```python
from build123d import *

# Parameters (mm, degrees)
SKETCH_1_R      = 1.2
EXTRUDE_1_DEPTH = 15
SKETCH_1_3_R    = 1.2
EXTRUDE_2_DEPTH = 15


with BuildPart() as part:
    # Sketch 1 → Extrude 1 (new body)
    with BuildSketch(Plane(origin=(0, 0, 0), x_dir=(1, 0, 0), z_dir=(0, 1, 0))):
        with BuildLine():
            Line((6.05, 2.5), (-6.05, 2.5))
            ThreePointArc((-6.05, 2.5), (-4.282233047, 1.767766953), (-3.55, 0))
            ThreePointArc((-3.55, 0), (-4.282233047, -1.767766953), (-6.05, -2.5))
            Line((-6.05, -2.5), (6.05, -2.5))
            ThreePointArc((6.05, -2.5), (8.55, 0), (6.05, 2.5))
        make_face()
        with Locations((6.05, 0)):
            Circle(SKETCH_1_R, mode=Mode.SUBTRACT)
        with BuildLine():
            ThreePointArc((-3.55, 0), (-4.282233047, 1.767766953), (-6.05, 2.5))
            ThreePointArc((-6.05, 2.5), (-8.55, 0), (-6.05, -2.5))
            ThreePointArc((-6.05, -2.5), (-4.282233047, -1.767766953), (-3.55, 0))
        make_face()
        with Locations((-6.05, 0)):
            Circle(SKETCH_1_R, mode=Mode.SUBTRACT)
    extrude(amount=EXTRUDE_1_DEPTH)

    # Sketch 1_3 → Extrude 2 (add)
    with BuildSketch(Plane(origin=(0, 0, 0), x_dir=(1, 0, 0), z_dir=(0, 1, 0))):
        with BuildLine():
            ThreePointArc((-3.55, 0), (-4.282233047, 1.767766953), (-6.05, 2.5))
            ThreePointArc((-6.05, 2.5), (-8.55, 0), (-6.05, -2.5))
            ThreePointArc((-6.05, -2.5), (-4.282233047, -1.767766953), (-3.55, 0))
        make_face()
        with Locations((-6.05, 0)):
            Circle(SKETCH_1_3_R, mode=Mode.SUBTRACT)
    extrude(amount=EXTRUDE_2_DEPTH)


solid = part.part
```
The listing builds one solid part. Answer for the finished solid, in the listing's coordinates (mm). Coordinates: 2 decimals unless noted, no trailing zeros. Loops run counter-clockwise (first coordinate to the right, second up) from the corner with the lowest first, then second, coordinate; pieces in that order, holes last. Notation, with made-up numbers: M 1,-26 L 38,-26 A20 cw 38,-20 Z; hole C 15.25,-37 d2. An arc over 180 degrees is marked long. Answer as a JSON object with one key per item and string values. Group by question number.
Item 1: Determine the mould class of faces 1 (the face through (0, 0, 0)), 2 (the face through (-7.25, 7.4, -0.05)), 3 (the face through (0, 7, -2.5)) for opening direction Z: +Z half, -Z half, draft (parallel to the pull), parting line (faces both ways), or undercut.
Item 2: Section C-C (x = -6.75) is taken. Write down the section's boundary in (y, z).
Item 3: Consider L1, parallel to X at y = 3.5, z = 0; L2, parallel to Z at x = -6.05, y = 4.25; L3, parallel to X at y = 1, z = 0.9. Determine where each line is inside the solid, lowest interval first.
Item 4: Section D-D (z = 2) is taken. Write down the section's boundary in (x, y).
Item 5: Section A-A (z = 0) is taken. Write down the section's boundary in (x, y).
Item 6: Section B-B (y = 14.25) is taken. Write down the section's boundary in (x, z).
Solved:
{
 "1": {"face 1": "draft", "face 2": "undercut", "face 3": "-Z half"},
 "2": {"outline": "M 0,-2.4 L 15,-2.4 L 15,-0.97 L 0,-0.97 Z; M 0,0.97 L 15,0.97 L 15,2.4 L 0,2.4 Z"},
 "3": {"L1": "x = -8.55 to -7.25, -4.85 to 4.85, 7.25 to 8.55", "L2": "z = -2.5 to -1.2, 1.2 to 2.5", "L3": "x = -8.38 to -6.84, -5.26 to 5.26, 6.84 to 8.38"},
 "4": {"outline": "M -7.55,0 L 7.55,0 L 7.55,15 L -7.55,15 Z"},
 "5": {"outline": "M -8.55,0 L -7.25,0 L -7.25,15 L -8.55,15 Z; M -4.85,0 L 4.85,0 L 4.85,15 L -4.85,15 Z; M 7.25,0 L 8.55,0 L 8.55,15 L 7.25,15 Z"},
 "6": {"outline": "M -6.05,-2.5 L 6.05,-2.5 A2.5 ccw 6.05,2.5 L -6.05,2.5 A2.5 ccw Z; hole C -6.05,0 d2.4; hole C 6.05,0 d2.4"}
}
